Input: part model. Units: mm. Frame: model coordinates. Face numbers are marked on the shaded views. A direction names the side the tool comes from. Coordinates: 2 decimals unless noted, no trailing zeros. Loops run counter-clockwise (first coordinate to the right, second up) from the corner with the lowest first, then second, coordinate; pieces in that order, holes last.
(1) Section A-A, the plane x = 0. Return loops of the section in (y, z), then the cut area to 3 significant figures.
(2) Contact query for flat-ended pins moving along their axis: P1, Ø7, axis at x = 0, y = 0, coming from the -Z side; P2, Ø3, axis at y = -5, z = 8.5, coming from the -X side; P3, Ø1.5, axis at y = 19, z = 9.5, coming from the -X side; P4, Ø6, axis at x = -15.5, y = 37, coming from the +Z side. Output: stop coordinate, or through.
(3) Set-up query: the marked faces 1, 2 and 3. Return all of +Z, -Z, +X, -X, +Y, -Y with unobstructed straight access to the full face (end or side cutting, diameter ignored); none if empty.
(4) Section C-C, the plane z = -8.5. Return loops of the section in (x, y).
(5) Line query: L1, parallel to Y at x = 0, z = -3.5; L2, parallel to Z at x = -25, y = 18; L3, parallel to Y at x = 0, z = 6.5. Output: solid intervals per line, ascending.
```python
from build123d import *

# Parameters (mm, degrees)
SKETCH1_R               = 63.5
BOSS_EXTRUDE1_DEPTH     = 11.90625
SKETCH2_R               = 11.90625
BOSS_EXTRUDE2_DEPTH     = 15.08125
CUT_EXTRUDE1_DEPTH      = 92.060112572
CUT_EXTRUDE1_DEPTH_BACK = 92.060112572
SKETCH3_R               = 3.96875
FILLET1_R               = 6.35


with BuildPart() as part:
    # Sketch1 → Boss-Extrude1 (new, symmetric)
    with BuildSketch(Plane.XY):
        Circle(SKETCH1_R)
    extrude(amount=BOSS_EXTRUDE1_DEPTH, both=True)

    # Sketch2 → Boss-Extrude2 (add, symmetric)
    with BuildSketch(Plane.XY):
        with Locations(Location((0, 0, 0), (0, 0, 180))):
            Circle(SKETCH2_R)
    extrude(amount=BOSS_EXTRUDE2_DEPTH, both=True)

    # Sketch3 → Cut-Extrude1 (cut, two sides: drawn at the far end of the back side and taken through both)
    with BuildSketch(Plane.XY.offset(-CUT_EXTRUDE1_DEPTH_BACK)):
        Circle(SKETCH3_R)
    extrude(amount=CUT_EXTRUDE1_DEPTH + CUT_EXTRUDE1_DEPTH_BACK, mode=Mode.SUBTRACT)

    # Fillet1
    # the kernel refuses this fillet: 6.35 mm, written as the material it adds along each edge
    with BuildSketch(Plane(origin=(0, 0, -11.90625), x_dir=(-1, 0, 0), z_dir=(0, 1, 0))) as fillet1_piece_1:
        with BuildLine():
            CenterArc((17.405511314, -6.35), FILLET1_R, 90, 60)
            Line((17.405511314, 0), (11.90625, 0))
            Line((11.90625, 0), (11.90625, -3.175))
        make_face()
    revolve(axis=Axis((0, 0, -11.90625), (0, 0, 1)))
    with BuildSketch(Plane(origin=(0, 0, 11.90625), x_dir=(-1, 0, 0), z_dir=(0, 1, 0))) as fillet1_piece_2:
        with BuildLine():
            CenterArc((17.405511314, 6.35), FILLET1_R, 210, 60)
            Line((11.90625, 3.175), (11.90625, 0))
            Line((11.90625, 0), (17.405511314, 0))
        make_face()
    revolve(axis=Axis((0, 0, 11.90625), (0, 0, 1)))
    # the kernel refuses this fillet: 6.35 mm, written as the material it takes off along each edge
    with BuildSketch(Plane(origin=(0, 0, -11.90625), x_dir=(1, 0, 0), z_dir=(0, -1, 0))) as fillet1_2_piece_1:
        with BuildLine():
            CenterArc((63.5 - FILLET1_R, FILLET1_R), FILLET1_R, 270, 90)
            Line((63.5 - FILLET1_R, 0), (63.5, 0))
            Line((63.5, 0), (63.5, FILLET1_R))
        make_face()
    revolve(axis=Axis((0, 0, -11.90625), (0, 0, 1)), mode=Mode.SUBTRACT)
    with BuildSketch(Plane(origin=(0, 0, 11.90625), x_dir=(1, 0, 0), z_dir=(0, -1, 0))) as fillet1_2_piece_2:
        with BuildLine():
            CenterArc((63.5 - FILLET1_R, -FILLET1_R), FILLET1_R, 0, 90)
            Line((63.5 - FILLET1_R, 0), (63.5, 0))
            Line((63.5, 0), (63.5, -FILLET1_R))
        make_face()
    revolve(axis=Axis((0, 0, 11.90625), (0, 0, 1)), mode=Mode.SUBTRACT)


solid = part.part
```
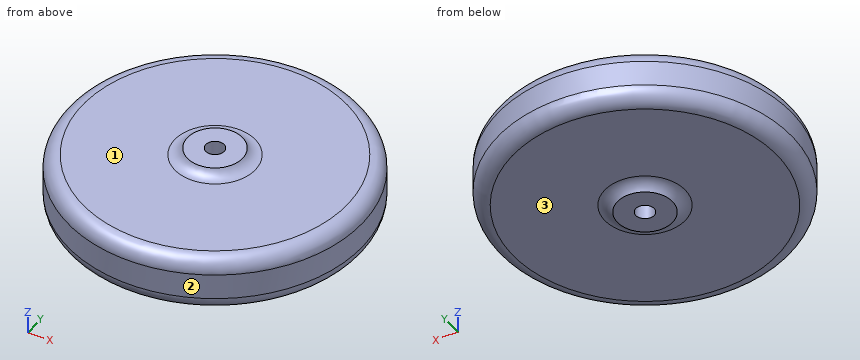
Report:
1. outline: (-63.5, -5.56) arc R6.35 ccw to (-57.15, -11.91) - (-17.41, -11.91) arc R6.35 cw to (-11.91, -15.08) - (-3.97, -15.08) - (-3.97, 15.08) - (-11.91, 15.08) arc R6.35 cw to (-17.41, 11.91) - (-57.15, 11.91) arc R6.35 ccw to (-63.5, 5.56) - close; (3.97, -15.08) - (11.91, -15.08) arc R6.35 cw to (17.41, -11.91) - (57.15, -11.91) arc R6.35 ccw to (63.5, -5.56) - (63.5, 5.56) arc R6.35 ccw to (57.15, 11.91) - (17.41, 11.91) arc R6.35 cw to (11.91, 15.08) - (3.97, 15.08) - close
1. area: 2,920 mm2
2. P1: passes through
2. P2: stops at x = -63.15
2. P3: stops at x = -59.74
2. P4: stops at z = 11.91
3. face 1: +Z
3. face 2: +Z, -Z
3. face 3: -Z
4. outline: circle Ø125.55 at (0, 0); hole circle Ø7.94 at (0, 0)
5. L1: y = -63.5 to -3.97, 3.97 to 63.5
5. L2: z = -11.91 to 11.91
5. L3: y = -63.43 to -3.97, 3.97 to 63.43
